The model under review builds one solid part; all positions refer to its coordinate system, in mm. A direction names the side the tool comes from. Round coordinates to 2 decimals unless told otherwise and drop trailing zeros. Write each loop counter-clockwise with the first axis right and the second up, starting at its lowest first coordinate (ties: lowest second). Pieces come first, ordered by that corner, then holes. Notation, with made-up numbers: (-12.75, -24.5) - (38.25, -24.5) arc R27 ccw to (38.25, -5.5) - close; hole circle Ø7 at (-30, 85). An arc over 180 degrees is marked (long way). One line per question, with ' | ' between items. Start each with the question number.
```python
from build123d import *

# Parameters (mm, degrees)
SKETCH2_R          = 1.65
CUT_EXTRUDE1_DEPTH = 10
SKETCH4_R          = 1.625
SKETCH4_R_2        = 3
SKETCH4_R_3        = 1.9
CUT_EXTRUDE2_DEPTH = 34.234018716
SKETCH4_3_R        = 3
CUT_EXTRUDE3_DEPTH = 34.234018857


with BuildPart() as part:
    # Sketch1 → Revolve1 (revolve)
    with BuildSketch(Plane.XY):
        Polygon((11.15, 20.4), (11.15, 70.35), (14.9, 70.35), (14.9, 27.8), (23.5, 18.8), (23.5, 0), (14.225, 0), (14.225, 20.4), align=None)
    revolve(axis=Axis((0, 0, 0), (0, 1, 0)))

    # Sketch2 → Cut-Extrude1 (cut)
    with BuildSketch(Plane.XZ):
        with Locations((0, 19.625)):
            Circle(SKETCH2_R)
        with Locations((0, -19.625)):
            Circle(SKETCH2_R)
        with Locations((-19.625, 0)):
            Circle(SKETCH2_R)
        with Locations((19.625, 0)):
            Circle(SKETCH2_R)
    extrude(amount=-CUT_EXTRUDE1_DEPTH, mode=Mode.SUBTRACT)

    # Sketch4 → Cut-Extrude2 (cut, through all)
    with BuildSketch(Plane(origin=(0, 0, 0), x_dir=(0, -1, 0), z_dir=(-0.707106781, 0, 0.707106781))):
        with Locations((-16.875, 0)):
            Circle(SKETCH4_R)
        with Locations((-62.35, 0)):
            Circle(SKETCH4_R_2)
        with Locations((-52.45, 0)):
            Circle(SKETCH4_R_3)
    extrude(amount=-CUT_EXTRUDE2_DEPTH, mode=Mode.SUBTRACT)

    # Sketch4_3 → Cut-Extrude3 (cut, through all)
    with BuildSketch(Plane(origin=(0, 0, 0), x_dir=(0, -1, 0), z_dir=(-0.707106781, 0, 0.707106781))):
        with Locations((-37.15, 0)):
            Circle(SKETCH4_3_R)
    extrude(amount=CUT_EXTRUDE3_DEPTH, mode=Mode.SUBTRACT)


solid = part.part
```
1. Add section B-B, the plane x = 0. Write out the cut boundary in (y, z) (3 decimals).
2. Add section A-A, the plane z = 0. Write out the cut boundary in (x, y) (3 decimals), then the cut area to 3 significant figures.
3. Add section C-C, the plane y = 64. Write out the cut boundary in (x, z).
4. Wall thickness on line 1 along Z through (x, y) = (0, 4.5) (3 decimals); line 2 along Z through (x, y) = (0, 13) (3 decimals); line 3 along Z through (x, y) = (0, 44): over which ranges is each line inside the solid? List them lowest first. Write a range as [from, to].
5. Machinability: for faces 1 (the face through (-20.934, 4.93, -1.004)), 2 (the face through (9.68, 59.49, -8.4)), 3 (the face through (14.21, 48.78, -4.48)), which of the approach directions +Z, -Z, +X, -X, +Y, -Y give a long, thin tool a straight path to every point of the face, cutting with its end or side? Answer none if there is none.
6. The part is to be moulded in two halves that separate along X. For faces 4 (the face through (9.54, 50.64, -8.73)), 5 (the face through (-0.21, 4.93, -17.99)), 6 (the face through (0, 0, 15)), 7 (the face through (-3.35, 27.24, 15.07)), say which applies: pulls with the +X half, pulls with the -X half, needs draft (parallel to the pull), parting line crosses it, or undercut.
7. Add section D-D, the plane x = -9. State how many separate pieces and enclosed holes the cut face has, then the cut area to 3 significant figures.
8. Clearance check with flat-ended pins moving along their axes: P1, Ø3, axis at x = -17.5, z = 10.5, coming from the +Y side; P2, Ø8, axis at y = 52.5, z = 16, coming from the +X side; P3, Ø14, axis at x = -3.5, z = -2, coming from the -Y side; P4, Ø3, axis at x = -19.625, z = 0, coming from the +Y side (3 decimals). State where each tip first meets the part, or that it passes through.
Geometry check:
1) outline: (0, -23.5) - (18.8, -23.5) - (27.8, -14.9) - (70.35, -14.9) - (70.35, -11.15) - (20.4, -11.15) - (20.4, -14.225) - (0, -14.225) - (0, -17.975) - (10, -17.975) - (10, -21.275) - (0, -21.275) - close; (0, 14.225) - (20.4, 14.225) - (20.4, 11.15) - (70.35, 11.15) - (70.35, 14.9) - (27.8, 14.9) - (18.8, 23.5) - (0, 23.5) - (0, 21.275) - (10, 21.275) - (10, 17.975) - (0, 17.975) - close
2) outline: (-23.5, 0) - (-21.275, 0) - (-21.275, 10) - (-17.975, 10) - (-17.975, 0) - (-14.225, 0) - (-14.225, 20.4) - (-11.15, 20.4) - (-11.15, 70.35) - (-14.9, 70.35) - (-14.9, 27.8) - (-23.5, 18.8) - close; (11.15, 20.4) - (14.225, 20.4) - (14.225, 0) - (17.975, 0) - (17.975, 10) - (21.275, 10) - (21.275, 0) - (23.5, 0) - (23.5, 18.8) - (14.9, 27.8) - (14.9, 70.35) - (11.15, 70.35) - close | area: 737 mm2
3) outline: (5.91, -9.45) arc R11.15 cw (long way) to (9.45, -5.91) - (12.16, -8.61) arc R14.9 ccw (long way) to (8.61, -12.16) - close
4) line 1: z = [-23.5, -21.275], [-17.975, -14.225], [14.225, 17.975], [21.275, 23.5] | line 2: z = [-23.5, -14.225], [14.225, 23.5] | line 3: z = [-14.9, -11.15], [11.15, 14.9]
5) face 1: -Y | face 2: none | face 3: +Y
6) face 4: undercut | face 5: undercut | face 6: needs draft | face 7: parting line crosses it
7) separate pieces: 3 | enclosed holes: 0 | area: 995 mm2
8) P1: stops at y = 23.61 | P2: stops at x = 8.83 | P3: passes through | P4: stops at y = 24.425
